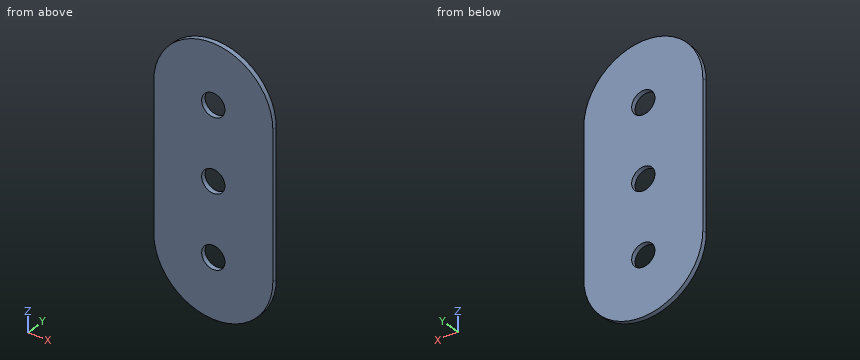
```python
from build123d import *

# Parameters (mm, degrees)
F0_R     = 2.54
F1_DEPTH = 1


with BuildPart() as f1:
    # F0 (on Front) → F1 (new body)
    with BuildSketch(Plane.XZ):
        with BuildLine():
            ThreePointArc((11.155105, 31.938435), (-1.844895, 18.938435), (-14.844895, 31.938435))
            Line((-14.844895, 31.938435), (-14.844895, -0.061565))
            ThreePointArc((-14.844895, -0.061565), (-1.844895, 12.938435), (11.155105, -0.061565))
            Line((11.155105, -0.061565), (11.155105, 31.938435))
        make_face()
        with Locations((-1.844895, 15.938435)):
            Circle(F0_R, mode=Mode.SUBTRACT)
        with BuildLine():
            ThreePointArc((11.155105, 31.938435), (-1.844895, 44.938435), (-14.844895, 31.938435))
            ThreePointArc((-14.844895, 31.938435), (-1.844895, 18.938435), (11.155105, 31.938435))
        make_face()
        with Locations((-1.844895, 31.938435)):
            Circle(F0_R, mode=Mode.SUBTRACT)
        with BuildLine():
            ThreePointArc((11.155105, -0.061565), (-1.844895, 12.938435), (-14.844895, -0.061565))
            ThreePointArc((-14.844895, -0.061565), (-1.844895, -13.061565), (11.155105, -0.061565))
        make_face()
        with Locations((-1.844895, -0.061565)):
            Circle(F0_R, mode=Mode.SUBTRACT)
    extrude(amount=F1_DEPTH)


solid = f1.part
```
For this review, take the finished solid that the model builds, in its own axes (mm). Give positions to 0.01 mm unless a question says otherwise; leave off trailing zeros. Write each loop counter-clockwise with the first axis right and the second up, starting at its lowest first coordinate (ties: lowest second). Pieces come first, ordered by that corner, then holes. Notation, with made-up numbers: M -32.5,75.25 L -9.5,75.25 A29 cw -9.5,102.25 Z; hole C 78,11 d1. An arc over 180 degrees is marked long. Answer as CSV lines item,"result".
1. Consider section C-C, the plane z = -2. Write out the cut boundary in (x, y), then the cut area to 3 significant figures.
Findings:
outline,"M -14.7,-1 L -3.49,-1 L -3.49,0 L -14.7,0 Z; M -0.2,-1 L 11.01,-1 L 11.01,0 L -0.2,0 Z"
area,"22.4 mm2"
2. Consider section A-A, the plane x = -2. Write out the cut boundary in (y, z).
Findings:
outline,"M -1,-13.06 L 0,-13.06 L 0,-2.6 L -1,-2.6 Z; M -1,2.47 L 0,2.47 L 0,13.4 L -1,13.4 Z; M -1,18.47 L 0,18.47 L 0,29.4 L -1,29.4 Z; M -1,34.47 L 0,34.47 L 0,44.94 L -1,44.94 Z"
3. Wall thickness on line 1 (Z direction, x = -1.75, y = -0.35); line 2 (Z direction, x = -3, y = -0.2); line 3 (Z direction, x = 7.25, y = -0.9): over which ranges is each line inside the solid? List them lowest first.
Findings:
line 1,"z = -13.06 to -2.6, 2.48 to 13.4, 18.48 to 29.4, 34.48 to 44.94"
line 2,"z = -13.01 to -2.32, 2.2 to 13.68, 18.2 to 29.68, 34.2 to 44.89"
line 3,"z = -9.35 to 41.23"
4. Consider section D-D, the plane x = 9. Write out the cut boundary in (y, z).
Findings:
outline,"M -1,-7.23 L 0,-7.23 L 0,39.11 L -1,39.11 Z"
5. For pin 1 (4 mm diameter, centred on x = -1.84, z = 15.94, fed in from -Y), flat-tipped, find the tip position at first contact; note if it passes through.
Findings:
pin 1,"passes through"
6. Consider section B-B, the plane y = -0.35. Write out the cut boundary in (x, z), then the cut area to 3 significant figures.
Findings:
outline,"M -14.84,-0.06 A13 ccw 11.16,-0.06 L 11.16,31.94 A13 ccw -14.84,31.94 Z; hole C -1.84,-0.06 d5.08; hole C -1.84,15.94 d5.08; hole C -1.84,31.94 d5.08"
area,"1,300 mm2"
